Part model, mm, in its own coordinate system. Face numbers are marked on the shaded views. A direction names the side the tool comes from. Round coordinates to 2 decimals unless told otherwise and drop trailing zeros. Write each loop counter-clockwise with the first axis right and the second up, starting at its lowest first coordinate (ties: lowest second). Pieces come first, ordered by that corner, then holes. Notation, with made-up numbers: (50.25, 1.5) -> (60.25, 1.5) arc R24 cw to (60.25, 34.5) -> close; hole circle Ø6 at (60, 82.5). An arc over 180 degrees is marked (long way). Return JSON: item names as keys, results as strings. Group by question number.
(1) Mould opens along Z. For the marked faces 1, 2, 3 and 4 say: +Z half, -Z half, draft (parallel to the pull), parting line (faces both ways), or undercut.
(2) Drop flat-ended pins along their axis: pin 1 Ø2 at (x, z) = (-3.5, 0.5) entering from -Y; pin 2 Ø0.6 at (x, y) = (9, 13) entering from +Z; pin 3 Ø1.6 at (x, y) = (9.5, 13) entering from -Z; pin 4 Ø1 at (x, y) = (4.5, 3) entering from +Z. Give the stop position or say it passes through.
(3) Drill centre lines: L1, parallel to Z at x = 0.25, y = 4.25; L2, parallel to X at y = 13.75, z = 0; L3, parallel to Y at x = 9.75, z = 0.5. Where is each one in solid material? Low to high. Write a range as from..to.
(4) Saw through at A-A (y = 5.25). List the corners of the cut face in (x, z).
(5) Saw through at C-C (x = 7.5). List the corners of the cut face in (y, z), plus the area to 3 significant figures.
(6) Saw through at B-B (z = 0). List the corners of the cut face in (x, y), plus the area to 3 significant figures.
(7) Saw through at D-D (y = 13.5). List the corners of the cut face in (x, z).
(8) Tool access for the marked faces 5, 6, 7 and 8: list every direction of +Z, -Z, +X, -X, +Y, -Y with a clear straight run to the whole face (end or side of a thin tool).
from build123d import *

# Parameters (mm, degrees)
EXTRUDE_1_DEPTH     = 9
EXTRUDE_1_2_DEPTH   = 9
EXTRUDE_2_DEPTH     = 6
SKETCH_7_W          = 5.379535364
SKETCH_7_H          = 3
EXTRUDE_3_DEPTH     = 5
FILLET_1_R          = 10
CHAMFER_1_SIZE      = 0.5
SKETCH_8_R          = 1.51
CUT_EXTRUDE_1_DEPTH = 3


with BuildPart() as part:
    # Sketch 4 → Extrude 1 (new body)
    with BuildSketch(Plane(origin=(0, 0, 0), x_dir=(1, 0, 0), z_dir=(0, 1, 0))):
        with BuildLine():
            Line((-5.326508943, 1.1), (4.991869226, 1.1))
            ThreePointArc((4.991869226, 1.1), (5.269632733, 1.184250756), (5.453789099, 1.408610265))
            Line((5.453789099, 1.408610265), (5.90531838, 2.498377946))
            ThreePointArc((5.90531838, 2.498377946), (5.933789047, 2.787323397), (5.796899922, 3.04337304))
            Line((5.796899922, 3.04337304), (3.766484258, 5.073191861))
            ThreePointArc((3.766484258, 5.073191861), (3.604290607, 5.181540331), (3.412982843, 5.219586503))
            Line((3.412982843, 5.219586503), (-2.466960198, 5.219586503))
            ThreePointArc((-2.466960198, 5.219586503), (-2.630617478, 5.19204422), (-2.776244778, 5.112451681))
            Line((-2.776244778, 5.112451681), (-5.905207067, 2.649164418))
            ThreePointArc((-5.905207067, 2.649164418), (-6.092318767, 2.31622196), (-5.989810106, 1.948317839))
            Line((-5.989810106, 1.948317839), (-5.326508943, 1.1))
        make_face()
    extrude(amount=EXTRUDE_1_DEPTH)



with BuildPart() as body_2:
    # Sketch 4 → Extrude 1 2 (new body)
    with BuildSketch(Plane(origin=(0, 0, 0), x_dir=(1, 0, 0), z_dir=(0, 1, 0))):
        with BuildLine():
            Line((3.766484258, -5.073191861), (5.796899922, -3.04337304))
            ThreePointArc((5.796899922, -3.04337304), (5.933789047, -2.787323397), (5.90531838, -2.498377946))
            Line((5.90531838, -2.498377946), (5.453789099, -1.408610265))
            ThreePointArc((5.453789099, -1.408610265), (5.269632733, -1.184250756), (4.991869226, -1.1))
            Line((4.991869226, -1.1), (-5.326508943, -1.1))
            Line((-5.326508943, -1.1), (-5.989810106, -1.948317839))
            ThreePointArc((-5.989810106, -1.948317839), (-6.092318767, -2.31622196), (-5.905207067, -2.649164418))
            Line((-5.905207067, -2.649164418), (-2.776244778, -5.112451681))
            ThreePointArc((-2.776244778, -5.112451681), (-2.630617478, -5.19204422), (-2.466960198, -5.219586503))
            Line((-2.466960198, -5.219586503), (3.412982843, -5.219586503))
            ThreePointArc((3.412982843, -5.219586503), (3.604290607, -5.181540331), (3.766484258, -5.073191861))
        make_face()
    extrude(amount=EXTRUDE_1_2_DEPTH)


with BuildPart() as part_1:
    add(part.part)

    add(body_2.part)  # Extrude 2 merges body 2
    # Sketch 5 → Extrude 2 (add)
    with BuildSketch(Plane(origin=(0, 9, 0), x_dir=(1, 0, 0), z_dir=(0, 1, 0))):
        with BuildLine():
            Line((3.766484258, -5.073191861), (5.796899922, -3.04337304))
            ThreePointArc((5.796899922, -3.04337304), (5.905324208, -2.881143349), (5.943398507, -2.689767682))
            Line((5.943398507, -2.689767682), (5.943398507, 2.689767682))
            ThreePointArc((5.943398507, 2.689767682), (5.905324208, 2.881143349), (5.796899922, 3.04337304))
            Line((5.796899922, 3.04337304), (3.766484258, 5.073191861))
            ThreePointArc((3.766484258, 5.073191861), (3.604290607, 5.181540331), (3.412982843, 5.219586503))
            Line((3.412982843, 5.219586503), (-2.466960198, 5.219586503))
            ThreePointArc((-2.466960198, 5.219586503), (-2.630617478, 5.19204422), (-2.776244778, 5.112451681))
            Line((-2.776244778, 5.112451681), (-5.905207067, 2.649164418))
            ThreePointArc((-5.905207067, 2.649164418), (-6.045723715, 2.474654122), (-6.095922486, 2.256299239))
            Line((-6.095922486, 2.256299239), (-6.095922486, -2.256299239))
            ThreePointArc((-6.095922486, -2.256299239), (-6.045723715, -2.474654122), (-5.905207067, -2.649164418))
            Line((-5.905207067, -2.649164418), (-2.776244778, -5.112451681))
            ThreePointArc((-2.776244778, -5.112451681), (-2.630617478, -5.19204422), (-2.466960198, -5.219586503))
            Line((-2.466960198, -5.219586503), (3.412982843, -5.219586503))
            ThreePointArc((3.412982843, -5.219586503), (3.604290607, -5.181540331), (3.766484258, -5.073191861))
        make_face()
    extrude(amount=EXTRUDE_2_DEPTH)

    # Sketch 7 → Extrude 3 (add)
    with BuildSketch(Plane(origin=(5.943398507, 0, 0), x_dir=(0, 0, -1), z_dir=(1, 0, 0))):
        with Locations((0, 13.5)):
            Rectangle(SKETCH_7_W, SKETCH_7_H)
    extrude(amount=EXTRUDE_3_DEPTH)

    # Fillet 1
    # the kernel refuses this fillet: 10 mm, written as the material it adds along each edge
    with BuildSketch(Plane(origin=(5.943398507, 12, -2.689767682), x_dir=(-0.38275133514604787, 0, -0.923851403334929), z_dir=(0, 1, 0))) as fillet_1_piece_1:
        with BuildLine():
            CenterArc((8.285757547, -6.127192899), FILLET_1_R, 142.213613886, 15.282174956)
            Line((-0.952756487, -2.299679547), (0, 0))
            ThreePointArc((0, 0), (0.191375668, -0.038074298), (0.382751335, 0))
        make_face()
    extrude(amount=3)
    with BuildSketch(Plane(origin=(5.943398507, 12, 2.689767682), x_dir=(-0.3827513351460759, 0, 0.9238514033349174), z_dir=(0, 1, 0))) as fillet_1_piece_2:
        with BuildLine():
            CenterArc((8.285757547, 6.127192899), FILLET_1_R, 202.504211157, 15.282174956)
            Line((-0.952756487, 2.299679547), (0, 0))
            ThreePointArc((0, 0), (0.191375668, 0.038074298), (0.382751335, 0))
        make_face()
    extrude(amount=3)

    # Chamfer 1
    chamfer_1_edges = [part_1.edges().sort_by_distance(p)[0] for p in [
        (10.943398507, 13.5, -2.689767682),
        (10.943398507, 13.5, 2.689767682),
    ]]
    chamfer(chamfer_1_edges, length=CHAMFER_1_SIZE)

    # Sketch 8 → Cut-Extrude 1 (cut)
    with BuildSketch(Plane(origin=(0, 15, 0), x_dir=(1, 0, 0), z_dir=(0, 1, 0))):
        with Locations(Location((8, 0, 0), (0, 0, 270))):
            Circle(SKETCH_8_R)
    extrude(amount=-CUT_EXTRUDE_1_DEPTH, mode=Mode.SUBTRACT)


solid = part_1.part
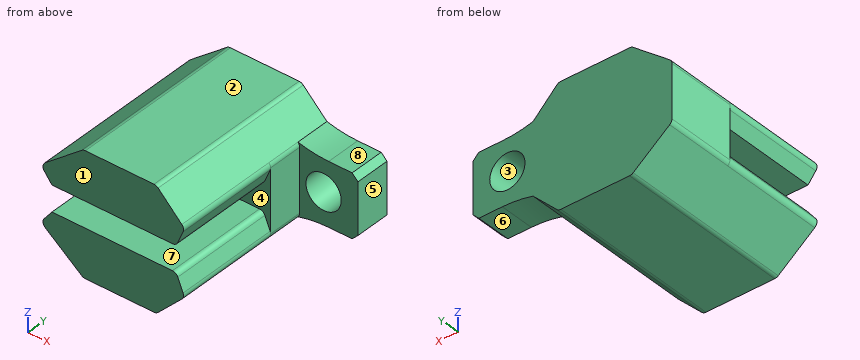
Computed values:
{
 "1": {"face 1": "draft", "face 2": "+Z half", "face 3": "undercut", "face 4": "undercut"},
 "2": {"pin 1": "y = 0", "pin 2": "z = 2.69", "pin 3": "z = -2.69", "pin 4": "z = 4.84"},
 "3": {"L1": "-5.22..-1.1, 1.1..5.22", "L2": "-6.1..6.49, 9.51..10.94", "L3": "12..15"},
 "4": {"outline": "(-5.99, -1.95) arc R0.5 ccw to (-5.91, -2.65) -> (-2.78, -5.11) arc R0.5 ccw to (-2.47, -5.22) -> (3.41, -5.22) arc R0.5 ccw to (3.77, -5.07) -> (5.8, -3.04) arc R0.5 ccw to (5.91, -2.5) -> (5.45, -1.41) arc R0.5 ccw to (4.99, -1.1) -> (-5.33, -1.1) -> close; (-5.99, 1.95) -> (-5.33, 1.1) -> (4.99, 1.1) arc R0.5 ccw to (5.45, 1.41) -> (5.91, 2.5) arc R0.5 ccw to (5.8, 3.04) -> (3.77, 5.07) arc R0.5 ccw to (3.41, 5.22) -> (-2.47, 5.22) arc R0.5 ccw to (-2.78, 5.11) -> (-5.91, 2.65) arc R0.5 ccw to start"},
 "5": {"outline": "(12, -2.73) -> (15, -2.73) -> (15, -1.42) -> (12, -1.42) -> close; (12, 1.42) -> (15, 1.42) -> (15, 2.73) -> (12, 2.73) -> close", "area": "7.85 mm2"},
 "6": {"outline": "(-6.1, 9) -> (5.94, 9) -> (5.94, 12) -> (6.49, 12) -> (6.49, 15) -> (-6.1, 15) -> close; (9.51, 12) -> (10.94, 12) -> (10.94, 15) -> (9.51, 15) -> close", "area": "78.2 mm2"},
 "7": {"outline": "(-6.1, -2.26) arc R0.5 ccw to (-5.91, -2.65) -> (-2.78, -5.11) arc R0.5 ccw to (-2.47, -5.22) -> (3.41, -5.22) arc R0.5 ccw to (3.77, -5.07) -> (5.8, -3.04) arc R10 cw to (8.43, -2.69) -> (10.44, -2.69) -> (10.94, -2.19) -> (10.94, 2.19) -> (10.44, 2.69) -> (8.43, 2.69) arc R10 cw to (5.8, 3.04) -> (3.77, 5.07) arc R0.5 ccw to (3.41, 5.22) -> (-2.47, 5.22) arc R0.5 ccw to (-2.78, 5.11) -> (-5.91, 2.65) arc R0.5 ccw to (-6.1, 2.26) -> close; hole circle Ø3.02 at (8, 0)"},
 "8": {"face 5": "+Z, -Z, +X, +Y, -Y", "face 6": "-Z, +X, +Y, -Y", "face 7": "+X, -X, -Y", "face 8": "+Z, +X, +Y, -Y"}
}
